Here's how the part is built. I have some questions about the finished solid (model axes, mm). A direction names the side the tool comes from. Give positions to 0.01 mm unless a question says otherwise; leave off trailing zeros. Loops run counter-clockwise (first coordinate to the right, second up) from the corner with the lowest first, then second, coordinate; pieces in that order, holes last.
Q1. Suppose I cut it at A-A (z = -30.5). List the corners of the cut face in (x, y) for me.
Q2. Suppose I cut it at D-D (y = 26). List the corners of the cut face in (x, z) for me.
Q3. I need wall thicknesses on probe 1 along X at (y, z) = (5.25, -70.5); probe 2 along Z at (x, y) = (-13, 27.75); probe 3 along Z at (x, y) = (-41.5, 9.5). Which ranges of each line are inside material? Lowest first, please.
Q4. For faces 4 (the face through (6.514, 18.663, -50.799)), 5 (the face through (-49, 10, -58)), 6 (the face through (1.34, 3.97, -55.89)), 7 (the face through (6, 30, -26)), 8 (the face through (-24, 25, -88)), which set-ups out of +Z, -Z, +X, -X, +Y, -Y let a thin tool reach every point of the face, with its end or its side?
Q5. Thinking about a two-plate mould opening in Z: for faces 1 (the face through (-22, 26, -89)), 2 (the face through (7, 9, -55.2)), 3 (the face through (-33.3, 5, 7)), which applies, pulls with the +Z half, pulls with the -Z half, needs draft (parallel to the pull), parting line crosses it, or undercut?
Q6. Suppose I cut it at B-B (x = -29). List the corners of the cut face in (y, z) for me, and give its area (3 significant figures).
Q7. I'm going to push flat-ended pins straight in: P1, Ø1, axis at x = -38.5, z = -27.5, coming from the +Y side; P2, Ø5.5, axis at x = -1, z = -0.5, coming from the +Y side; P3, Ø14, axis at x = -14, y = 12.5, coming from the -Z side. Where does each tip first touch, or does it pass through?
Q8. Suppose I cut it at C-C (x = -49). List the corners of the cut face in (y, z) for me.
Autodesk Inventor part; units mm, degrees
sketch "Sketch1" plane through (0, 0, 0) normal (0, 1, 0) x (-1, 0, 0)
  point P0 (0, 0)
sketch "Sketch2" plane through (0, 0, 0) normal (0, 1, 0) x (-1, 0, 0)
  circle A0 centre (0, 0) radius 1.25
  line L0 (60.55, 0) -> (-11.55, 0)
  line L1 (0, -71.35) -> (0, 13.35)
  circle A1 centre (49, 0) radius 1.25
  circle A2 centre (0, -58) radius 1.25
  circle A3 centre (49, -58) radius 1.25
  dimension "d0" = 2.5
  dimension "d3" = 49
  dimension "d6" = 58
extrude "Extrusion1" add sketch "Sketch2" along normal blind 10
sketch "Sketch3" plane through (0, 0, 0) normal (0, 1, 0) x (-1, 0, 0)
  line L0 (52.5, 3.5) -> (-3.5, 3.5)
  line L1 (-3.5, 3.5) -> (-3.5, -85)
  line L2 (-3.5, -85) -> (52.5, -85)
  line L3 (52.5, -85) -> (52.5, 3.5)
  circle A0 centre (49, 0) radius 1.25
  circle A1 centre (49, -58) radius 1.25
  circle A2 centre (0, 0) radius 1.25
  circle A3 centre (0, -58) radius 1.25
  line L4 (54.5, 5.5) -> (-5.5, 5.5)
  line L5 (-5.5, 5.5) -> (-5.5, -87)
  line L6 (-5.5, -87) -> (54.5, -87)
  line L7 (54.5, -87) -> (54.5, 5.5)
  dimension "d11" = 3.5
  dimension "d12" = 27
  dimension "d13" = 3.5
  dimension "d14" = 3.5
  dimension "d15" = 2
extrude "Extrusion2" add sketch "Sketch3" along normal blind 2 contours L3 L2 L1 L0 | L7 L6 L5 L4
sketch "Sketch5" plane through (0, 0, 0) normal (0, 0, 1) x (1, 0, 0)
  line L0 (-54.5, 0) -> (5.5, 0)
  line L1 (5.5, 0) -> (5.5, 2)
  line L2 (-54.5, 2) -> (5.5, 2)
  line L3 (-54.5, 0) -> (-54.5, 2)
  line L4 (5.5, 0) -> (7.5, 0)
  line L5 (7.5, 0) -> (7.5, 30)
  line L6 (7.5, 30) -> (5.5, 30)
  line L7 (5.5, 30) -> (5.5, 0)
  point P0 (0, 0)
  dimension "d18" = 2
  dimension "d19" = 30
sketch3d "3D Sketch1"
sketch3d "3D Sketch2"
  line L0 (5.5, 2, -87) -> (5.5, 2, 5.5)
  line L1 (5.5, 2, 5.5) -> (-54.5, 2, 5.5)
  line L2 (-54.5, 2, 5.5) -> (-54.5, 2, -87)
sweep "Sweep2" add profiles "Sketch5" path "3D Sketch2" contours L1 L7 L6 L5 L4
sketch "Sketch6" plane through (7.5, 0, -87) normal (0, 0, -1) x (-1, 0, 0)
  line L0 (2, 30) -> (62, 30)
  line L1 (2, 30) -> (2, 2)
  line L2 (2, 25) -> (62, 25)
  line L3 (62, 30) -> (62, 2)
  line L4 (2, 25) -> (2, 2)
  line L5 (2, 2) -> (62, 2)
  line L6 (2, 2) -> (62, 2)
  line L7 (62, 25) -> (62, 2)
  line L8 (0, 0) -> (0, 30)
  line L9 (0, 30) -> (2, 30)
  line L10 (64, 0) -> (0, 0)
  line L11 (64, 0) -> (64, 30)
  line L12 (64, 30) -> (62, 30)
  point P0 (7.5, 0)
  dimension "d25" = 5
extrude "Extrusion3" add sketch "Sketch6" along normal blind 2 contours L0 L3 L2 L1 | L1 L5 L3 L12 L11 L10 L8 L9
sketch "Sketch8" plane through (-56.5, 30, 7.5) normal (0, 0, 1) x (1, 0, 0)
  line L0 (64, -30) -> (0, -30)
  line L1 (0, -30) -> (0, 0)
  line L2 (64, -30) -> (64, 0)
  point P0 (56.5, -30)
  point P1 (20, -30)
sketch "Sketch9" plane through (0, 2, 0) normal (0, 1, 0) x (1, 0, 0)
  circle A0 centre (0, 0) radius 1.25
  circle A1 centre (0, 0) radius 1.25
  circle A2 centre (-49, 0) radius 1.25
  circle A3 centre (-49, 0) radius 1.25
  circle A4 centre (-49, 58) radius 1.25
  circle A5 centre (-49, 58) radius 1.25
  circle A6 centre (0, 58) radius 1.25
  circle A7 centre (0, 58) radius 1.25
  circle A8 centre (0, 58) radius 1.25
  circle A9 centre (0, 0) radius 2.5
  circle A10 centre (-49, 0) radius 1.25
  circle A11 centre (-49, 0) radius 2.5
  circle A12 centre (0, 58) radius 2.5
  circle A13 centre (-49, 58) radius 2.5
  dimension "d44" = 5
  dimension "d45" = 5
  dimension "d46" = 5
  dimension "d47" = 5
extrude "Extrusion6" add sketch "Sketch9" along normal blind 4
sketch "Sketch11" plane through (7.5, 0, 7.5) normal (1, 0, 0) x (0, 0, -1)
  line L0 (7.5, -6) -> (7.5, 36)
  point P0 (7.5, 0)
ref_plane "Work Plane1" through (0, 2, 2.5) normal (0, 0, 1) x (1, 0, 0)
ref_plane "Work Plane2" through (0, 2, 2.8) normal (0, 0, 1) x (1, 0, 0)
sketch "Sketch12" plane through (7.5, 0, 7.5) normal (1, 0, 0) x (0, 0, -1)
  line L0 (7.5, -6) -> (7.5, 36)
  line L1 (4.7, -6) -> (4.7, 36)
  line L2 (13.1008, 0) -> (18.181, 0)
  line L3 (96.5, 0) -> (0, 0)
  point P0 (7.5, 0)
  dimension "d51" = 0
ref_plane "Work Plane3" through (-49, 6, -58) normal (0, 1, 0) x (1, 0, 0)
sketch "Sketch13" plane through (7.5, 0, 7.5) normal (1, 0, 0) x (0, 0, -1)
  line L0 (-19.3, 6) -> (115.8, 6)
  line L1 (10.8, 4.5) -> (19.8, 4.5)
  line L2 (19.8, 4.5) -> (19.8, 11)
  line L3 (19.8, 11) -> (10.8, 11)
  line L4 (10.8, 11) -> (10.8, 4.5)
  line L5 (28.2, 4.5) -> (45.2, 4.5)
  line L6 (45.2, 4.5) -> (45.2, 15)
  line L7 (45.2, 15) -> (28.2, 15)
  line L8 (28.2, 15) -> (28.2, 4.5)
  line L9 (4.7, -6) -> (4.7, 36)
  line L10 (53.7, 4.5) -> (62.7, 4.5)
  line L11 (62.7, 4.5) -> (62.7, 14.1644)
  line L12 (53.7, 14.1644) -> (53.7, 4.5)
  arc A0 (62.7, 14.1644) -> (53.7, 14.1644) centre (58.2, 14.1644) ccw
  point P0 (7.5, 0)
  point P1 (15.3, 11)
  point P2 (36.7, 15)
  dimension "d54" = 1.5
  dimension "d55" = 9
  dimension "d57" = 10.6
  dimension "d58" = 32
  dimension "d60" = 17
  dimension "d61" = 1.5
  dimension "d63" = 9
  dimension "d64" = 53.5
  dimension "d65" = 1.5
  dimension "d66" = 9
  dimension "d67" = 5
extrude "Extrusion7" cut sketch "Sketch13" against normal up to surface (2 mm away)
ref_plane "Work Plane5" through (2.7, 2, 0) normal (-1, 0, 0) x (0, -1, 0)
ref_plane "Work Plane4" through (2.5, 2, 0) normal (-1, 0, 0) x (0, -1, 0)
sketch "Sketch15" plane through (-56.5, 30, 7.5) normal (0, 0, 1) x (1, 0, 0)
  line L0 (59.2, -36) -> (59.2, 6)
  line L1 (-12.8, -24) -> (76.8, -24)
  line L2 (23.2, -22.5) -> (38.2, -22.5)
  line L3 (38.2, -22.5) -> (38.2, -28)
  line L4 (38.2, -28) -> (23.2, -28)
  line L5 (23.2, -28) -> (23.2, -22.5)
  point P0 (56.5, -30)
  dimension "d71" = 21
  dimension "d72" = 36
  dimension "d73" = 4
  dimension "d74" = 1.5
extrude "Extrusion8" cut sketch "Sketch15" against normal up to surface (2 mm away)
properties part number "PI_Skal"
Solutions:
1. outline: (-56.5, 0) - (7.5, 0) - (7.5, 4.5) - (5.5, 4.5) - (5.5, 2) - (-54.5, 2) - (-54.5, 30) - (-56.5, 30) - close; (5.5, 15) - (7.5, 15) - (7.5, 30) - (5.5, 30) - close
2. outline: (-56.5, -89) - (7.5, -89) - (7.5, 7.5) - (-56.5, 7.5) - close; hole (-54.5, -87) - (5.5, -87) - (5.5, 5.5) - (-54.5, 5.5) - close
3. probe 1: x = -56.5 to -54.5, 5.5 to 7.5
3. probe 2: z = -89 to -87, 5.5 to 7.5
3. probe 3: z = 5.5 to 7.5
4. face 4: +X
4. face 5: -Z, +Y
4. face 6: +Y
4. face 7: +Z, -Z, +X, -X, +Y
4. face 8: -Z
5. face 1: pulls with the -Z half
5. face 2: undercut
5. face 3: needs draft
6. outline: (0, -89) - (2, -89) - (2, 7.5) - (0, 7.5) - close; (7.5, 5.5) - (30, 5.5) - (30, 7.5) - (7.5, 7.5) - close; (25, -89) - (30, -89) - (30, -87) - (25, -87) - close
6. area: 248 mm2
7. P1: stops at y = 2
7. P2: stops at y = 10
7. P3: stops at z = 5.5
8. outline: (0, -89) - (2, -89) - (2, -60.5) - (6, -60.5) - (6, -59.25) - (10, -59.25) - (10, -56.75) - (6, -56.75) - (6, -55.5) - (2, -55.5) - (2, -2.5) - (6, -2.5) - (6, -1.25) - (10, -1.25) - (10, 1.25) - (6, 1.25) - (6, 2.5) - (2, 2.5) - (2, 5.5) - (30, 5.5) - (30, 7.5) - (0, 7.5) - close; (25, -89) - (30, -89) - (30, -87) - (25, -87) - close
